Could you check a few things on this model? Use its own coordinates, in mm. Give positions to 0.01 mm unless a question says otherwise; leave off trailing zeros. Loops run counter-clockwise (first coordinate to the right, second up) from the corner with the lowest first, then second, coordinate; pieces in that order, holes last.
1. Imagine slicing it at C-C (x = 17). List the corners of the cut face in (y, z) for me.
2. Imagine slicing it at D-D (y = 7). List the corners of the cut face in (x, z) for me, plus the area to 3 significant figures.
3. I need wall thicknesses on line 1 along X through (y, z) = (0.5, 1); line 2 along X through (y, z) = (3, 0.45). Which ranges of each line are inside material? Lowest first, please.
4. Imagine slicing it at A-A (x = 27). List the corners of the cut face in (y, z) for me, plus the area to 3 significant figures.
```python
from build123d import *

# Parameters (mm, degrees)
F0_W     = 87
F0_H     = 55
F1_DEPTH = 2.8
F2_W     = 60
F2_H     = 18
F3_DEPTH = 25
F4_R     = 8.99999


# Not quite as in the source:
# - a fillet or chamfer is up to 0.001 mm smaller than in the source, because OpenCascade refuses the exact size


with BuildPart() as f1:
    # F0 (on Top) → F1 (new body)
    with BuildSketch(Plane.XY):
        Rectangle(F0_W, F0_H)
    extrude(amount=F1_DEPTH)

    # F2 (on face) → F3 (cut)
    with BuildSketch(Plane.XY.offset(2.8)):
        with Locations((43.5, 0)):
            Rectangle(F2_W, F2_H)
    extrude(amount=-F3_DEPTH, mode=Mode.SUBTRACT)

    # F4 (radius 9 in the source; OpenCascade refuses exactly that, so slightly less here)
    f4_edges = [f1.edges().sort_by_distance(p)[0] for p in [
        (13.5, 9, 1.4),
        (13.5, -9, 1.4),
    ]]
    fillet(f4_edges, radius=F4_R)


solid = f1.part
```
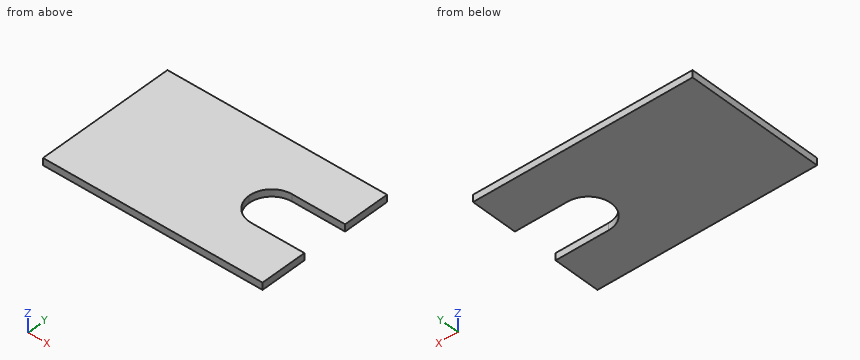
Derived:
1. outline: (-27.5, 0) - (-7.12, 0) - (-7.12, 2.8) - (-27.5, 2.8) - close; (7.12, 0) - (27.5, 0) - (27.5, 2.8) - (7.12, 2.8) - close
2. outline: (-43.5, 0) - (16.84, 0) - (16.84, 2.8) - (-43.5, 2.8) - close
2. area: 169 mm2
3. line 1: x = -43.5 to 13.51
3. line 2: x = -43.5 to 14.01
4. outline: (-27.5, 0) - (-9, 0) - (-9, 2.8) - (-27.5, 2.8) - close; (9, 0) - (27.5, 0) - (27.5, 2.8) - (9, 2.8) - close
4. area: 104 mm2
